Can you work these out from the model? Positions are in its coordinate system, mm. A direction names the side the tool comes from. Round coordinates to 2 decimals unless told otherwise and drop trailing zeros. Order: outer loops, then holes, each group sorted by start corner. A loop starts at its lowest first (then second) coordinate and runs counter-clockwise, first axis right, second up. Notation, with made-up numbers: (-10.5, -16) -> (-2.5, -16) arc R19 ccw to (-2.5, -5) -> close; hole circle Ø7 at (55.25, 61). An arc over 180 degrees is marked (long way). Use a Markdown table: item, result. Add a question column.
Q1. If we section it at A-A on y = 10: List the corners of the cut face in (x, z) for me, plus the area to 3 significant figures.
Q2. We'd pull the mould along X, two halves only. Please class faces 1 (the face through (-4.336, -19.524, 7.395)), 2 (the face through (0, -2, 18)), 3 (the face through (-1.5, -11, 1)): +X half, -X half, draft (parallel to the pull), parting line (faces both ways), or undercut.
Q3. I'm going to push flat-ended pins straight in: pin 1 Ø8 at (x, y) = (-8.5, 0.5) entering from +Z; pin 2 Ø1 at (y, z) = (-1.5, 13) entering from +X (3 decimals); pin 3 Ø2 at (y, z) = (-10.5, 0.5) entering from -X. Where does each tip first touch, or does it pass through?
Q4. If we section it at C-C on x = 0: List the corners of the cut face in (y, z) for me, plus the area to 3 significant figures.
Q5. If we section it at D-D on z = 14: List the corners of the cut face in (x, y) for me, plus the area to 3 significant figures.
Q6. For faces 4 (the face through (3.233, -1.341, 9.888)), 5 (the face through (-7.9, -8.32, 0.99)), 6 (the face through (0, 0, 0)), which set-ups out of +Z, -Z, +X, -X, +Y, -Y let a thin tool reach every point of the face, with its end or its side?
Q7. If we section it at B-B on x = -6.5: List the corners of the cut face in (y, z) for me, plus the area to 3 significant figures.
Q8. I need wall thicknesses on line 1 along Y through (x, z) = (0, 10.25); line 2 along X through (y, z) = (-3, 14.25); line 3 along Z through (x, y) = (-6, 17). Which ranges of each line are inside material? Lowest first, please. Write a range as [from, to].
```python
from build123d import *

# Parameters (mm, degrees)
F0_R     = 20
F1_DEPTH = 15
F2_R     = 18
F3_DEPTH = 13
F5_R     = 3.5
F5_R_2   = 1.5
F6_DEPTH = 16
F8_DEPTH = 2


with BuildPart() as f1:
    # F0 (on Top) → F1 (new body)
    with BuildSketch(Plane.XY):
        Circle(F0_R)
    extrude(amount=F1_DEPTH)

    # F2 (on face) → F3 (cut)
    with BuildSketch(Plane.XY.offset(15)):
        Circle(F2_R)
    extrude(amount=-F3_DEPTH, mode=Mode.SUBTRACT)

    # F5 (on face) → F6 (join)
    with BuildSketch(Plane.XY.offset(2)):
        Circle(F5_R)
        Circle(F5_R_2, mode=Mode.SUBTRACT)
    extrude(amount=F6_DEPTH)

    # F7 (on Top) → F8 (cut)
    with BuildSketch(Plane.XY):
        with BuildLine():
            ThreePointArc((-9.3298084702, -15.3933321249), (-5.5623058987, -17.1190172933), (-1.5, -17.9373911147))
            Line((-1.5, -17.9373911147), (-1.5, -4.6165253058))
            Line((-1.5, -4.6165253058), (-9.3298084702, -15.3933321249))
        make_face()
        with BuildLine():
            Line((9.3298084702, -15.3933321249), (1.5, -4.6165253058))
            Line((1.5, -4.6165253058), (1.5, -17.9373911147))
            ThreePointArc((1.5, -17.9373911147), (5.5623058987, -17.1190172933), (9.3298084702, -15.3933321249))
        make_face()
        with BuildLine():
            Line((16.5959472134, -6.9695434636), (3.9270509831, -2.8531695489))
            Line((3.9270509831, -2.8531695489), (11.7568594534, -13.6299763681))
            ThreePointArc((11.7568594534, -13.6299763681), (14.5623058987, -10.5801345413), (16.5959472134, -6.9695434636))
        make_face()
        with BuildLine():
            Line((17.5229981965, 4.1163739147), (4.8541019662, 0))
            Line((4.8541019662, 0), (17.5229981965, -4.1163739147))
            ThreePointArc((17.5229981965, -4.1163739147), (17.8803518916, -2.071959515), (18, 0))
            ThreePointArc((18, 0), (17.8803518916, 2.071959515), (17.5229981965, 4.1163739147))
        make_face()
        with BuildLine():
            Line((11.7568594534, 13.6299763681), (3.9270509831, 2.8531695489))
            Line((3.9270509831, 2.8531695489), (16.5959472134, 6.9695434636))
            ThreePointArc((16.5959472134, 6.9695434636), (14.5623058987, 10.5801345413), (11.7568594534, 13.6299763681))
        make_face()
        with BuildLine():
            Line((1.5, 17.9373911147), (1.5, 4.6165253058))
            Line((1.5, 4.6165253058), (9.3298084702, 15.3933321249))
            ThreePointArc((9.3298084702, 15.3933321249), (5.5623058987, 17.1190172933), (1.5, 17.9373911147))
        make_face()
        with BuildLine():
            Line((-1.5, 4.6165253058), (-1.5, 17.9373911147))
            ThreePointArc((-1.5, 17.9373911147), (-5.5623058987, 17.1190172933), (-9.3298084702, 15.3933321249))
            Line((-9.3298084702, 15.3933321249), (-1.5, 4.6165253058))
        make_face()
        with BuildLine():
            Line((-3.9270509831, 2.8531695489), (-11.7568594534, 13.6299763681))
            ThreePointArc((-11.7568594534, 13.6299763681), (-14.5623058987, 10.5801345413), (-16.5959472134, 6.9695434636))
            Line((-16.5959472134, 6.9695434636), (-3.9270509831, 2.8531695489))
        make_face()
        with BuildLine():
            Line((-4.8541019662, 0), (-17.5229981965, 4.1163739147))
            ThreePointArc((-17.5229981965, 4.1163739147), (-18, 0), (-17.5229981965, -4.1163739147))
            Line((-17.5229981965, -4.1163739147), (-4.8541019662, 0))
        make_face()
        with BuildLine():
            ThreePointArc((-16.5959472134, -6.9695434636), (-14.5623058987, -10.5801345413), (-11.7568594534, -13.6299763681))
            Line((-11.7568594534, -13.6299763681), (-3.9270509831, -2.8531695489))
            Line((-3.9270509831, -2.8531695489), (-16.5959472134, -6.9695434636))
        make_face()
    extrude(amount=F8_DEPTH, mode=Mode.SUBTRACT)


solid = f1.part
```
Answer below:
| question | item | result |
|---|---|---|
| 1 | outline | (-17.32, 0) -> (-14.97, 0) -> (-14.97, 15) -> (-17.32, 15) -> close; (-9.12, 0) -> (-5.41, 0) -> (-5.41, 2) -> (-9.12, 2) -> close; (-1.5, 0) -> (1.5, 0) -> (1.5, 2) -> (-1.5, 2) -> close; (5.41, 0) -> (9.12, 0) -> (9.12, 2) -> (5.41, 2) -> close; (14.97, 0) -> (17.32, 0) -> (17.32, 15) -> (14.97, 15) -> close |
| 1 | area | 91.4 mm² |
| 2 | face 1 | parting line |
| 2 | face 2 | draft |
| 2 | face 3 | undercut |
| 3 | pin 1 | z = 2 |
| 3 | pin 2 | x = 19.975 |
| 3 | pin 3 | x = -17.6 |
| 4 | outline | (-20, 0) -> (20, 0) -> (20, 15) -> (18, 15) -> (18, 2) -> (3.5, 2) -> (3.5, 18) -> (1.5, 18) -> (1.5, 2) -> (-1.5, 2) -> (-1.5, 18) -> (-3.5, 18) -> (-3.5, 2) -> (-18, 2) -> (-18, 15) -> (-20, 15) -> close |
| 4 | area | 196 mm² |
| 5 | outline | circle Ø40 at (0, 0); circle Ø7 at (0, 0); hole circle Ø36 at (0, 0); hole circle Ø3 at (0, 0) |
| 5 | area | 270 mm² |
| 6 | face 4 | +Z |
| 6 | face 5 | +Z, -Z |
| 6 | face 6 | -Z, +X, -X, +Y, -Y |
| 7 | outline | (-18.91, 0) -> (-16.79, 0) -> (-16.79, 15) -> (-18.91, 15) -> close; (-11.5, 0) -> (-6.39, 0) -> (-6.39, 2) -> (-11.5, 2) -> close; (-3.69, 0) -> (-0.53, 0) -> (-0.53, 2) -> (-3.69, 2) -> close; (0.53, 0) -> (3.69, 0) -> (3.69, 2) -> (0.53, 2) -> close; (6.39, 0) -> (11.5, 0) -> (11.5, 2) -> (6.39, 2) -> close; (16.79, 0) -> (18.91, 0) -> (18.91, 15) -> (16.79, 15) -> close |
| 7 | area | 96.9 mm² |
| 8 | line 1 | [-20, -18], [-3.5, -1.5], [1.5, 3.5], [18, 20] |
| 8 | line 2 | [-19.77, -17.75], [-1.8, 1.8], [17.75, 19.77] |
| 8 | line 3 | [0, 15] |
